Build history of the part. All positions in model axes, mm. Face numbers are marked on the shaded views. A direction names the side the tool comes from. Round coordinates to 2 decimals unless told otherwise and drop trailing zeros. Order: outer loops, then holes, each group sorted by start corner. A loop starts at its lowest first (then second) coordinate and runs counter-clockwise, first axis right, second up. Notation, with made-up numbers: M 24.5,9.5 L 32.5,9.5 A17 ccw 32.5,42.5 Z; hole C -18.5,-23 d9. An arc over 180 degrees is marked long. One line per question, with ' | ' between items. Start each with the question number.
from build123d import *

# Parameters (mm, degrees)
SKETCH_1_W                   = 40
SKETCH_1_H                   = 66.7
EXTRUDE_1_DEPTH              = 2
SKETCH_2_W                   = 4
SKETCH_2_H                   = 66.7
EXTRUDE_2_DEPTH              = 100
CUT_EXTRUDE_1_DEPTH          = 115.526077816
CUT_EXTRUDE_1_DEPTH_BACK     = 115.526077816
HOLE_WIZARD_M4_1_D           = 3.3
HOLE_WIZARD_M4_1_CSINK_D     = 4.05
HOLE_WIZARD_M4_1_CSINK_ANGLE = 90
HOLE_WIZARD_M4_2_AT_2_COUNT  = 2
HOLE_WIZARD_M4_2_AT_2_PITCH  = 68.59294731
HOLE_WIZARD_M4_2_AT_3_COUNT  = 2
HOLE_WIZARD_M4_2_AT_3_PITCH  = 26
HOLE_WIZARD_M4_2_AT_4_COUNT  = 2
HOLE_WIZARD_M4_2_AT_4_PITCH  = 62.376998966
HOLE_WIZARD_M4_2_AT_5_COUNT  = 2
HOLE_WIZARD_M4_2_AT_5_PITCH  = 56.7
SKETCH_11_W                  = 66.7
SKETCH_11_H                  = 2
EXTRUDE_3_DEPTH              = 100
SKETCH_13_W                  = 40
SKETCH_13_H                  = 66.7
EXTRUDE_4_DEPTH              = 2
SKETCH_14_W                  = 4
SKETCH_14_H                  = 66.7
EXTRUDE_5_DEPTH              = 100
CUT_EXTRUDE_2_DEPTH          = 180.589037806
CUT_EXTRUDE_2_DEPTH_BACK     = 180.589037806
HOLE_WIZARD_M4_3_AT_2_COUNT  = 2
HOLE_WIZARD_M4_3_AT_2_PITCH  = 26
HOLE_WIZARD_M4_3_AT_3_COUNT  = 2
HOLE_WIZARD_M4_3_AT_3_PITCH  = 62.376998966
HOLE_WIZARD_M4_3_AT_4_COUNT  = 2
HOLE_WIZARD_M4_3_AT_4_PITCH  = 56.7
CUT_EXTRUDE_3_REACH          = 181.589
SKETCH_18_R                  = 9.5
CUT_EXTRUDE_4_REACH          = 181.589
SKETCH_21_R                  = 11
CUT_EXTRUDE_5_REACH          = 181.589
SKETCH_22_R                  = 4.5
FILLET_1_R                   = 2
CUT_EXTRUDE_6_REACH          = 193.604
SKETCH_23_W                  = 36
SKETCH_23_H                  = 66.7
CUT_EXTRUDE_7_REACH          = 164.752
SKETCH_24_W                  = 36
SKETCH_24_H                  = 66.7
HOLE_WIZARD_M3_1_D           = 2.5
HOLE_WIZARD_M3_1_CSINK_D     = 3.05
HOLE_WIZARD_M3_1_CSINK_ANGLE = 90


with BuildPart() as part:
    # Sketch 1 → Extrude 1 (new body)
    with BuildSketch(Plane(origin=(0, 0, 0), x_dir=(1, 0, 0), z_dir=(0, 1, 0))):
        Rectangle(SKETCH_1_W, SKETCH_1_H)
    extrude(amount=EXTRUDE_1_DEPTH)

    # Sketch 2 → Extrude 2 (add)
    with BuildSketch(Plane(origin=(0, 2, 0), x_dir=(1, 0, 0), z_dir=(0, 1, 0))):
        with Locations((-18, 0)):
            Rectangle(SKETCH_2_W, SKETCH_2_H)
    extrude(amount=EXTRUDE_2_DEPTH)

    # Sketch 5 → Cut-Extrude 1 (cut, two sides: drawn at the far end of the back side and taken through both)
    with BuildSketch(Plane.ZY.offset(20).offset(-CUT_EXTRUDE_1_DEPTH_BACK)):
        with BuildLine():
            ThreePointArc((0, 102), (23.582011153, 92.232011153), (33.35, 68.65))
            Line((33.35, 68.65), (33.35, 102))
            Line((33.35, 102), (0, 102))
        make_face()
        with BuildLine():
            ThreePointArc((-33.35, 68.65), (-23.582011153, 92.232011153), (0, 102))
            Line((0, 102), (-33.35, 102))
            Line((-33.35, 102), (-33.35, 68.65))
        make_face()
    extrude(amount=CUT_EXTRUDE_1_DEPTH + CUT_EXTRUDE_1_DEPTH_BACK, mode=Mode.SUBTRACT)

    # Hole Wizard M4 _1 (through all)
    with Locations(Plane.ZY.offset(20)):
        with Locations((0, 97.65), (25.11473671, 54.15), (-25.11473671, 54.15)):
            CounterSinkHole(HOLE_WIZARD_M4_1_D / 2, HOLE_WIZARD_M4_1_CSINK_D / 2, counter_sink_angle=HOLE_WIZARD_M4_1_CSINK_ANGLE)

    # Sketch 10 → Hole Wizard M4 _2 (revolve, cut)
    with BuildSketch(Plane(origin=(15, 2, -28.35), x_dir=(0, 0, 1), z_dir=(1, 0, 0))):
        Polygon((0, 0), (0, 2), (1.65, 2), (1.65, 0.375), (2.025, 0), align=None)
    hole_wizard_m4_2 = revolve(axis=Axis((15, 8.35, -28.35), (0, -1, 0)), mode=Mode.SUBTRACT)

    # Hole Wizard M4 _2 at 2: Hole Wizard M4 _2 ×2
    with Locations(*[Vector(-0.9508085645250022, 0, 0.3097790722852413) * (i * HOLE_WIZARD_M4_2_AT_2_PITCH) for i in range(1, HOLE_WIZARD_M4_2_AT_2_COUNT)]):
        add(hole_wizard_m4_2, mode=Mode.SUBTRACT)

    # Hole Wizard M4 _2 at 3: Hole Wizard M4 _2 ×2
    with Locations(*[(-i * HOLE_WIZARD_M4_2_AT_3_PITCH, 0, 0) for i in range(1, HOLE_WIZARD_M4_2_AT_3_COUNT)]):
        add(hole_wizard_m4_2, mode=Mode.SUBTRACT)

    # Hole Wizard M4 _2 at 4: Hole Wizard M4 _2 ×2
    with Locations(*[Vector(-0.4168203092647413, 0, 0.9089889052042635) * (i * HOLE_WIZARD_M4_2_AT_4_PITCH) for i in range(1, HOLE_WIZARD_M4_2_AT_4_COUNT)]):
        add(hole_wizard_m4_2, mode=Mode.SUBTRACT)

    # Hole Wizard M4 _2 at 5: Hole Wizard M4 _2 ×2
    with Locations(*[(0, 0, i * HOLE_WIZARD_M4_2_AT_5_PITCH) for i in range(1, HOLE_WIZARD_M4_2_AT_5_COUNT)]):
        add(hole_wizard_m4_2, mode=Mode.SUBTRACT)

    # Sketch 11 → Extrude 3 (add)
    with BuildSketch(Plane.ZY.offset(20)):
        with Locations((0, 16)):
            Rectangle(SKETCH_11_W, SKETCH_11_H)
    extrude(amount=EXTRUDE_3_DEPTH)



with BuildPart() as body_2:
    # Sketch 13 → Extrude 4 (new body)
    with BuildSketch(Plane(origin=(0, 0, 0), x_dir=(1, 0, 0), z_dir=(0, 1, 0))):
        with Locations((-140, 0)):
            Rectangle(SKETCH_13_W, SKETCH_13_H)
    extrude(amount=EXTRUDE_4_DEPTH)


with BuildPart() as part_1:
    add(part.part)

    add(body_2.part)  # Extrude 5 merges body 2
    # Sketch 14 → Extrude 5 (add)
    with BuildSketch(Plane(origin=(0, 2, 0), x_dir=(1, 0, 0), z_dir=(0, 1, 0))):
        with Locations((-122, 0)):
            Rectangle(SKETCH_14_W, SKETCH_14_H)
    extrude(amount=EXTRUDE_5_DEPTH)

    # Sketch 15 → Cut-Extrude 2 (cut, two sides: drawn at the far end of the back side and taken through both)
    with BuildSketch(Plane.ZY.offset(124).offset(-CUT_EXTRUDE_2_DEPTH_BACK)):
        with BuildLine():
            ThreePointArc((0, 102), (23.582011153, 92.232011153), (33.35, 68.65))
            Line((33.35, 68.65), (33.35, 102))
            Line((33.35, 102), (0, 102))
        make_face()
        with BuildLine():
            ThreePointArc((-33.35, 68.65), (-23.582011153, 92.232011153), (0, 102))
            Line((0, 102), (-33.35, 102))
            Line((-33.35, 102), (-33.35, 68.65))
        make_face()
    extrude(amount=CUT_EXTRUDE_2_DEPTH + CUT_EXTRUDE_2_DEPTH_BACK, mode=Mode.SUBTRACT)

    # Sketch 17 → Hole Wizard M4 _3 (revolve, cut)
    with BuildSketch(Plane(origin=(-129, 2, -28.35), x_dir=(0, 0, 1), z_dir=(1, 0, 0))):
        Polygon((0, 0), (0, 2), (1.65, 2), (1.65, 0.375), (2.025, 0), align=None)
    hole_wizard_m4_3 = revolve(axis=Axis((-129, 8.35, -28.35), (0, -1, 0)), mode=Mode.SUBTRACT)

    # Hole Wizard M4 _3 at 2: Hole Wizard M4 _3 ×2
    with Locations(*[(-i * HOLE_WIZARD_M4_3_AT_2_PITCH, 0, 0) for i in range(1, HOLE_WIZARD_M4_3_AT_2_COUNT)]):
        add(hole_wizard_m4_3, mode=Mode.SUBTRACT)

    # Hole Wizard M4 _3 at 3: Hole Wizard M4 _3 ×2
    with Locations(*[Vector(-0.41682030926474106, 0, 0.9089889052042636) * (i * HOLE_WIZARD_M4_3_AT_3_PITCH) for i in range(1, HOLE_WIZARD_M4_3_AT_3_COUNT)]):
        add(hole_wizard_m4_3, mode=Mode.SUBTRACT)

    # Hole Wizard M4 _3 at 4: Hole Wizard M4 _3 ×2
    with Locations(*[(0, 0, i * HOLE_WIZARD_M4_3_AT_4_PITCH) for i in range(1, HOLE_WIZARD_M4_3_AT_4_COUNT)]):
        add(hole_wizard_m4_3, mode=Mode.SUBTRACT)

    # Sketch 18 → Cut-Extrude 3 (cut, up to next)
    with BuildSketch(Plane.ZY.offset(124), mode=Mode.PRIVATE) as cut_extrude_3_sk1:
        with Locations((0, 68.65)):
            Circle(SKETCH_18_R)
    cut_extrude_3_tool1 = extrude(cut_extrude_3_sk1.sketch, amount=-CUT_EXTRUDE_3_REACH, mode=Mode.PRIVATE) & part_1.part
    add(cut_extrude_3_tool1.solids().sort_by_distance((-124, 68.65, 0))[0], mode=Mode.SUBTRACT)

    # Sketch 21 → Cut-Extrude 4 (cut, up to next)
    with BuildSketch(Plane(origin=(-16, 0, 0), x_dir=(0, 0, -1), z_dir=(1, 0, 0)), mode=Mode.PRIVATE) as cut_extrude_4_sk1:
        with Locations((0, 68.65)):
            Circle(SKETCH_21_R)
    cut_extrude_4_tool1 = extrude(cut_extrude_4_sk1.sketch, amount=-CUT_EXTRUDE_4_REACH, mode=Mode.PRIVATE) & part_1.part
    add(cut_extrude_4_tool1.solids().sort_by_distance((-16, 68.65, 0))[0], mode=Mode.SUBTRACT)

    # Sketch 22 → Cut-Extrude 5 (cut, up to next)
    with BuildSketch(Plane(origin=(-16, 0, 0), x_dir=(0, 0, -1), z_dir=(1, 0, 0)), mode=Mode.PRIVATE) as cut_extrude_5_sk1:
        with Locations((16.670989023, 59.025)):
            Circle(SKETCH_22_R)
    cut_extrude_5_tool1 = extrude(cut_extrude_5_sk1.sketch, amount=-CUT_EXTRUDE_5_REACH, mode=Mode.PRIVATE) & part_1.part
    add(cut_extrude_5_tool1.solids().sort_by_distance((-16, 59.025, -16.670989))[0], mode=Mode.SUBTRACT)

    # Fillet 1
    fillet_1_edges = [part_1.edges().sort_by_distance(p)[0] for p in [
        (-160, 1, -33.35),
        (-160, 1, 33.35),
        (20, 1, 33.35),
        (20, 1, -33.35),
    ]]
    fillet(fillet_1_edges, radius=FILLET_1_R)

    # Sketch 23 → Cut-Extrude 6 (cut, up to next)
    with BuildSketch(Plane(origin=(0, 2, 0), x_dir=(1, 0, 0), z_dir=(0, 1, 0)), mode=Mode.PRIVATE) as cut_extrude_6_sk1:
        with Locations((-142, 0)):
            Rectangle(SKETCH_23_W, SKETCH_23_H)
    cut_extrude_6_tool1 = extrude(cut_extrude_6_sk1.sketch, amount=-CUT_EXTRUDE_6_REACH, mode=Mode.PRIVATE) & part_1.part
    add(cut_extrude_6_tool1.solids().sort_by_distance((-142, 2, 0))[0], mode=Mode.SUBTRACT)

    # Sketch 24 → Cut-Extrude 7 (cut, up to next)
    with BuildSketch(Plane(origin=(0, 2, 0), x_dir=(1, 0, 0), z_dir=(0, 1, 0)), mode=Mode.PRIVATE) as cut_extrude_7_sk1:
        with Locations((2, 0)):
            Rectangle(SKETCH_24_W, SKETCH_24_H)
    cut_extrude_7_tool1 = extrude(cut_extrude_7_sk1.sketch, amount=-CUT_EXTRUDE_7_REACH, mode=Mode.PRIVATE) & part_1.part
    add(cut_extrude_7_tool1.solids().sort_by_distance((2, 2, 0))[0], mode=Mode.SUBTRACT)

    # Hole Wizard M3 _1 (through all)
    with Locations(Plane(origin=(-16, 0, 0), x_dir=(0, 0, -1), z_dir=(1, 0, 0))):
        with Locations((9, 6), (-9, 6)):
            CounterSinkHole(HOLE_WIZARD_M3_1_D / 2, HOLE_WIZARD_M3_1_CSINK_D / 2, counter_sink_angle=HOLE_WIZARD_M3_1_CSINK_ANGLE)


solid = part_1.part
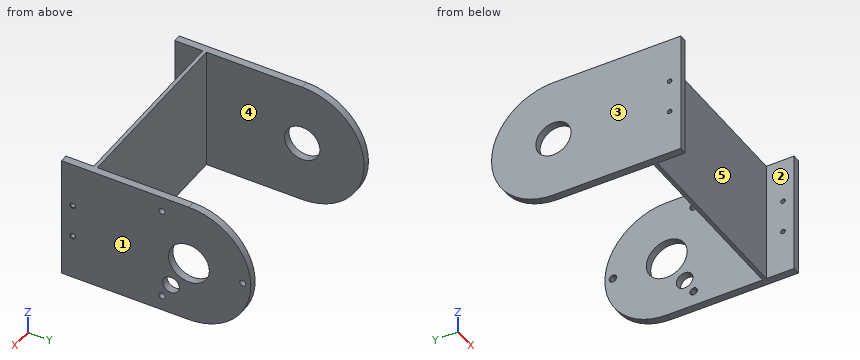
Item 1: Two-plate mould, pull along X, no slides. Class the marked faces 1, 2 and 3: +X half, -X half, draft (parallel to the pull), parting line (faces both ways), or undercut.
Item 2: Tool access for the marked faces 4 and 5: list every direction of +Z, -Z, +X, -X, +Y, -Y with a clear straight run to the whole face (end or side of a thin tool).
Item 3: Cut at B-B on z = -5.5. Write the cut outline in (x, y), then the cut area to 3 significant figures.
Item 4: Cut at D-D on x = -80. Write the cut outline in (y, z), then the cut area to 3 significant figures.
Item 5: Flat gauge pins, fed straight in: pin 1 (1.5 mm diameter, centred on y = 6, z = 9, fed in from +X); pin 2 (12 mm diameter, centred on x = -70, z = 3, fed in from +Y); pin 3 (4 mm diameter, centred on y = 6, z = 9, fed in from -X); pin 4 (3 mm diameter, centred on y = 6, z = -9, fed in from +X) (3 decimals). Where does each tip first touch, or does it go through?
Item 6: Wall check: line 1 along Z through (x, y) = (-17, 54); line 2 along Z through (x, y) = (-17, 6); line 3 along Y through (x, z) = (-17, 0). Give the ranges that are in metal, low to high. Write a range as [from, to].
Item 7: Cut at A-A on y = 97.65. Write the cut outline in (x, z) (3 decimals).
Item 8: Cut at C-C on y = 70. Write the cut outline in (x, z).
Results found:
1) face 1: +X half | face 2: undercut | face 3: -X half
2) face 4: +Z, -Z, +Y | face 5: +Z, -Z, -Y
3) outline: M -124,0 L -120,0 L -120,15 L -20,15 L -20,0 L -16,0 L -16,59.12 L -20,59.12 L -20,17 L -120,17 L -120,60.9 L -124,60.9 Z; M -124,76.4 L -120,76.4 L -120,101.54 L -124,101.54 Z; M -20,78.18 L -16,78.18 L -16,101.54 L -20,101.54 Z | area: 874 mm^2
4) outline: M 15,-33.35 L 17,-33.35 L 17,33.35 L 15,33.35 Z | area: 133 mm^2
5) pin 1: passes through | pin 2: stops at y = 17 | pin 3: stops at x = -124 | pin 4: stops at x = -16.025
6) line 1: z = [-33.35, -26.76], [-23.47, 23.47], [26.76, 33.35] | line 2: z = [-33.35, -10.25], [-7.75, 7.75], [10.25, 33.35] | line 3: y = [0, 57.65], [79.65, 96], [99.3, 102]
7) outline: M -124,-16.469 L -120,-16.469 L -120,16.469 L -124,16.469 Z; M -20,-16.469 L -16,-16.469 L -16,-1.65 L -19.625,-1.65 L -20,-2.025 Z; M -20,2.025 L -19.625,1.65 L -16,1.65 L -16,16.469 L -20,16.469 Z
8) outline: M -124,-33.32 L -120,-33.32 L -120,-9.4 L -124,-9.4 Z; M -124,9.4 L -120,9.4 L -120,33.32 L -124,33.32 Z; M -20,-33.32 L -16,-33.32 L -16,-10.92 L -20,-10.92 Z; M -20,10.92 L -16,10.92 L -16,33.32 L -20,33.32 Z
